Geometry: final body of the model. Coordinates: model frame, mm. A direction names the side the tool comes from. Give positions to 0.01 mm unless a question says otherwise; leave off trailing zeros. Loops run counter-clockwise (first coordinate to the right, second up) from the corner with the lowest first, then second, coordinate; pieces in that order, holes last. Notation, with made-up numbers: (-4, 78) -> (20, 78) arc R22 cw to (20, 101) -> close; hole circle Ø11 at (-12.5, 52). An arc over 180 degrees is marked (long way). Answer in a Markdown table with one row per item. Add a question column.
1) Line query: line 1 (Z direction, x = 30, y = -78.5); line 2 (Z direction, x = 73, y = 32); line 3 (Z direction, x = 134.5, y = 93.5) (3 decimals). Output: solid intervals per line, ascending. Write a range as from..to.
2) Draft query along Z for faces 3 (the flat face through (125, -1, 0)), 4 (the flat face through (190.95, -1.42, 99.3)), 5 (the flat face through (78.311, -24, 106.367)). Return one class per face: +Z half, -Z half, draft (parallel to the pull), parting line (faces both ways), or undercut.
3) Section query D-D (y = 27). Return the cut outline in (x, z).
4) Section query B-B (z = 42). Return the cut outline in (x, y), plus the area to 3 significant figures.
5) Section query C-C (x = 62). Return the cut outline in (y, z).
6) Access query for faces 1 (the flat face through (77, -1, 50.8)), 2 (the flat face through (151, 101.6, 70)). Directions: +Z, -Z, +X, -X, +Y, -Y. A direction counts if a zero-diameter tool reaches every point of the face in a straight line with its end or side. Return the directions, or none.
7) First-contact query: P1, Ø5, axis at x = 203.5, y = -59.5, coming from the +Z side; P2, Ø4, axis at x = 151.5, y = -4.5, coming from the +Z side; P3, Ø1, axis at y = -68.5, z = 103.5, coming from the +X side. Flat tips, straight axial feed; report the tip coordinate or a pass-through.
8) Section query A-A (y = 66.5). Return the cut outline in (x, z), plus the area to 3 significant figures.
```python
from build123d import *

# Parameters (mm, degrees)
F1_DEPTH = 101.6
F2_R     = 38.1
F3_DEPTH = 74.422
F5_DEPTH = 72.136


with BuildPart() as f1:
    # F0 (on Front) → F1 (new body, symmetric)
    with BuildSketch(Plane.XZ):
        Polygon((0, 50.8), (0, 0), (254, 0), (254, 50.8), (88.9, 177.8), (50.8, 127), (152.4, 50.8), (76.2, 50.8), align=None)
    extrude(amount=F1_DEPTH, both=True)

    # F2 (on face) → F3 (cut)
    with BuildSketch(Plane(origin=(118.9739776952, 0, 154.6661710037), x_dir=(0.7926239891, 0, -0.6097107608), z_dir=(0.6097107608, 0, 0.7926239891))):
        with Locations((30.880294776, 0)):
            Circle(F2_R)
    extrude(amount=-F3_DEPTH, mode=Mode.SUBTRACT)

    # F4 (on face) → F5 (cut)
    with BuildSketch(Plane(origin=(0, 0, 0), x_dir=(1, 0, 0), z_dir=(0, 0, -1))):
        Polygon((0, -50.8), (0, -101.6), (50.8, -101.6), align=None)
        Polygon((0, 101.6), (0, 50.8), (50.8, 101.6), align=None)
    extrude(amount=-F5_DEPTH, mode=Mode.SUBTRACT)


solid = f1.part
```
Evaluation:
| question | item | result |
|---|---|---|
| 1 | line 1 | 0..50.8 |
| 1 | line 2 | 0..50.8, 110.35..156.6 |
| 1 | line 3 | 0..50.8, 64.225..142.723 |
| 2 | face 3 | -Z half |
| 2 | face 4 | +Z half |
| 2 | face 5 | undercut |
| 3 | outline | (0, 0) -> (254, 0) -> (254, 50.8) -> (164.76, 119.45) -> (126.75, 70.04) -> (152.4, 50.8) -> (0, 50.8) -> close; (50.8, 127) -> (83.74, 102.3) -> (122.14, 152.23) -> (88.9, 177.8) -> close |
| 4 | outline | (0, -50.8) -> (50.8, -101.6) -> (254, -101.6) -> (254, 101.6) -> (50.8, 101.6) -> (0, 50.8) -> close |
| 4 | area | 49,000 mm² |
| 5 | outline | (-101.6, 0) -> (101.6, 0) -> (101.6, 50.8) -> (-101.6, 50.8) -> close; (-101.6, 118.6) -> (101.6, 118.6) -> (101.6, 141.93) -> (-101.6, 141.93) -> close |
| 6 | face 1 | -X, +Y, -Y |
| 6 | face 2 | +Z, -Z, +X, -X, +Y |
| 7 | P1 | z = 91.57 |
| 7 | P2 | z = 86.88 |
| 7 | P3 | x = 186.14 |
| 8 | outline | (15.7, 0) -> (254, 0) -> (254, 50.8) -> (88.9, 177.8) -> (50.8, 127) -> (152.4, 50.8) -> (15.7, 50.8) -> close |
| 8 | area | 22,600 mm² |
